Can you work these out from the model? Positions are in its coordinate system, mm. A direction names the side the tool comes from. Round coordinates to 2 decimals unless told otherwise and drop trailing zeros. Loops run counter-clockwise (first coordinate to the right, second up) from the corner with the lowest first, then second, coordinate; pieces in that order, holes last.
from build123d import *

# Parameters (mm, degrees)
F0_W     = 210
F0_H     = 100
F1_DEPTH = 76.2
F2_W     = 133
F2_H     = 64
F3_DEPTH = 76.201
F4_R     = 6.35
F5_R     = 20
F6_DEPTH = 100.001
F8_DEPTH = 100.001


with BuildPart() as f1:
    # F0 (on Front) → F1 (new body)
    with BuildSketch(Plane.XZ):
        with Locations((105, 50)):
            Rectangle(F0_W, F0_H)
    extrude(amount=F1_DEPTH)

    # F2 (on face) → F3 (cut, through all)
    with BuildSketch(Plane.XZ.offset(76.2)):
        with Locations((143.5, 50)):
            Rectangle(F2_W, F2_H)
    extrude(amount=-F3_DEPTH, mode=Mode.SUBTRACT)

    # F4
    f4_edges = [f1.edges().sort_by_distance(p)[0] for p in [
        (77, -38.1, 82),
        (77, -38.1, 18),
    ]]
    fillet(f4_edges, radius=F4_R)

    # F5 (on face) → F6 (cut, through all)
    with BuildSketch(Plane.XY.offset(100)):
        Polygon((190, 16.513776), (190, 0), (210, -20), (210, -56.2), (190, -76.2), (190, -91.743216), (258.705469, -91.743216), (258.705469, 16.513776), align=None)
        with Locations((170, -38.1)):
            Circle(F5_R)
    extrude(amount=-F6_DEPTH, mode=Mode.SUBTRACT)

    # F7 (on face) → F8 (cut, through all)
    with BuildSketch(Plane.XY.offset(100)):
        Polygon((65, -66.2), (0, -66.2), (0, -76.2), (75, -76.2), align=None)
    extrude(amount=-F8_DEPTH, mode=Mode.SUBTRACT)


solid = f1.part
(1) For faces 5 (the flat face through (146, -39, 82)), 6 (the flat face through (33, -66.2, 51)), 7 (the flat face through (0, -33, 49)), which set-ups out of +Z, -Z, +X, -X, +Y, -Y let a thin tool reach every point of the face, with its end or its side?
Worked answers:
face 5: +X, +Y, -Y
face 6: +Z, -Z, -X, -Y
face 7: +Z, -Z, -X, +Y, -Y
(2) If we mould it in two halves opening along Z, with no side actions, what happens to faces 1 (the flat face through (104, -38, 0)), 2 (the cylindrical face through (78.81, -37.57, 19.91)), 3 (the flat face through (73, 0, 51)), 4 (the cylindrical face through (78.91, -37.57, 80.19))? For each: released by +Z, released by -Z, zero draft, split by the parting line, or undercut.
Worked answers:
face 1: released by -Z
face 2: undercut
face 3: zero draft
face 4: undercut
(3) If we section it at C-C, the plane y = -38.1: List the corners of the cut face in (x, z) for me, then the cut area to 3 significant figures.
Worked answers:
outline: (0, 0) - (150, 0) - (150, 18) - (83.35, 18) arc R6.35 cw to (77, 24.35) - (77, 75.65) arc R6.35 cw to (83.35, 82) - (150, 82) - (150, 100) - (0, 100) - close; (190, 0) - (210, 0) - (210, 18) - (190, 18) - close; (190, 82) - (210, 82) - (210, 100) - (190, 100) - close
area: 11,100 mm2
(4) Will these pins go through, and if not, where does the flat tip stop? P1, Ø5, axis at x = 185, y = -33.5, coming from the -Z side; P2, Ø1, axis at y = -54, z = 69.5, coming from the +X side; P3, Ø19.5, axis at x = 27, z = 32.5, coming from the -Y side.
Worked answers:
P1: passes through
P2: stops at x = 77
P3: stops at y = -66.2
(5) If we section it at D-D, the plane y = -61.5: List the corners of the cut face in (x, z) for me, then the cut area to 3 significant figures.
Worked answers:
outline: (0, 0) - (204.7, 0) - (204.7, 18) - (83.35, 18) arc R6.35 cw to (77, 24.35) - (77, 75.65) arc R6.35 cw to (83.35, 82) - (204.7, 82) - (204.7, 100) - (0, 100) - close
area: 12,300 mm2
(6) If we section it at A-A, the plane x = 170: List the corners of the cut face in (y, z) for me, then the cut area to 3 significant figures.
Worked answers:
outline: (-76.2, 0) - (-58.1, 0) - (-58.1, 18) - (-76.2, 18) - close; (-76.2, 82) - (-58.1, 82) - (-58.1, 100) - (-76.2, 100) - close; (-18.1, 0) - (0, 0) - (0, 18) - (-18.1, 18) - close; (-18.1, 82) - (0, 82) - (0, 100) - (-18.1, 100) - close
area: 1,300 mm2
(7) If we section it at B-B, the plane z = 91.5: List the corners of the cut face in (x, y) for me, then the cut area to 3 significant figures.
Worked answers:
outline: (0, -66.2) - (65, -66.2) - (75, -76.2) - (190, -76.2) - (210, -56.2) - (210, -20) - (190, 0) - (0, 0) - close; hole circle Ø40 at (170, -38.1)
area: 13,600 mm2
(8) If I drill on line 1 (Y direction, x = 170, z = 6); line 2 (Z direction, x = 98.5, y = -5); line 3 (X direction, y = -38, z = 86), over which ranges is the centre line in solid material (lowest first)?
Worked answers:
line 1: y = -76.2 to -58.1, -18.1 to 0
line 2: z = 0 to 18, 82 to 100
line 3: x = 0 to 150, 190 to 210
